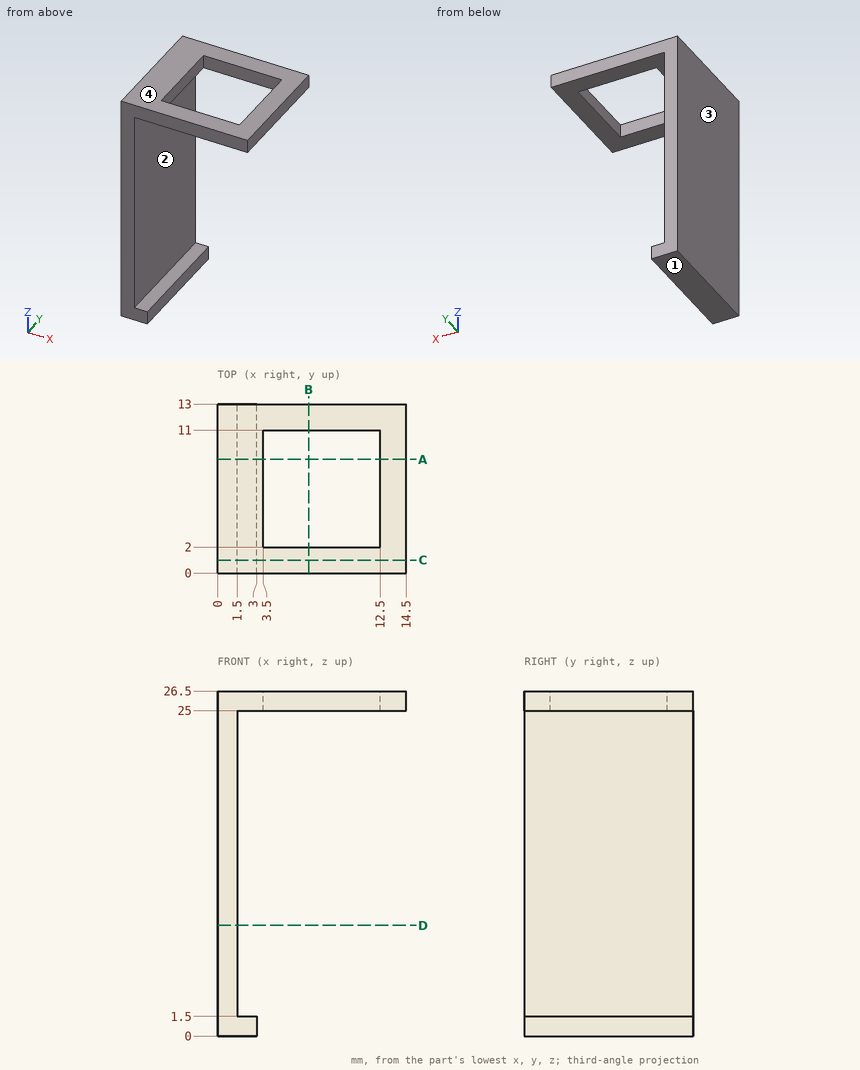
Check sheet for the drawn part. Datum: minimum x, y, z corner. Units: mm. Round coordinates to 2 decimals unless told otherwise and drop trailing zeros. Order: outer loops, then holes, each group sorted by start corner. A loop starts at its lowest first (then second) coordinate and runs counter-clockwise, first axis right, second up.
(1) Cross-section at C-C, the plane y = 1. Enter the section's corners in (x, z), and give its area (3 significant figures).
(2) Go/stop test with a flat-tipped pin: P1, Ø0.8, axis at y = 5, z = 1, coming from the +X side. Record where the tip stops, or that it passes through.
(3) Cross-section at B-B, the plane x = 7. Enter the section's corners in (y, z), and give its area (3 significant figures).
(4) Cross-section at D-D, the plane z = 8.5. Enter the section's corners in (x, y), and give its area (3 significant figures).
(5) Scan lines: probe 1 along Z at (x, y) = (2.75, 11.75); probe 2 along X at (y, z) = (5.25, 13.5); probe 3 along Z at (x, y) = (13.25, 8.5). Record each from-to range of solid material in increasing order.
(6) Cross-section at A-A, the plane y = 8.75. Enter the section's corners in (x, z), and give its area (3 significant figures).
(7) Draft check along Z on the marked faces 1, 2, 3 and 4. Enter one of: pulls with the +Z half, pulls with the -Z half, needs draft (parallel to the pull), parting line crosses it, or undercut.
Check sheet entries:
1. outline: (0, 0) - (3, 0) - (3, 1.5) - (1.5, 1.5) - (1.5, 25) - (14.5, 25) - (14.5, 26.5) - (0, 26.5) - close
1. area: 61.5 mm2
2. P1: stops at x = 3
3. outline: (0, 25) - (2, 25) - (2, 26.5) - (0, 26.5) - close; (11, 25) - (13, 25) - (13, 26.5) - (11, 26.5) - close
3. area: 6.00 mm2
4. outline: (0, 0) - (1.5, 0) - (1.5, 13) - (0, 13) - close
4. area: 19.5 mm2
5. probe 1: z = 0 to 1.5, 25 to 26.5
5. probe 2: x = 0 to 1.5
5. probe 3: z = 25 to 26.5
6. outline: (0, 0) - (3, 0) - (3, 1.5) - (1.5, 1.5) - (1.5, 25) - (3.5, 25) - (3.5, 26.5) - (0, 26.5) - close; (12.5, 25) - (14.5, 25) - (14.5, 26.5) - (12.5, 26.5) - close
6. area: 48.0 mm2
7. face 1: pulls with the -Z half
7. face 2: undercut
7. face 3: needs draft
7. face 4: pulls with the +Z half
